from build123d import *

# Parameters (mm, degrees)
SKETCH1_W               = 131
SKETCH1_H               = 106
BOSS_EXTRUDE1_DEPTH     = 5
SKETCH6_R               = 2
CUT_EXTRUDE1_DEPTH      = 4
SKETCH7_R               = 1.4
CUT_EXTRUDE2_DEPTH      = 2.8
MIRROR2_COPY_1_SKETCH_R = 2
MIRROR2_COPY_1_DEPTH    = 4
MIRROR2_COPY_2_SKETCH_R = 1.4
MIRROR2_COPY_2_DEPTH    = 2.8
SKETCH10_W              = 40
SKETCH10_H              = 66
CUT_EXTRUDE5_DEPTH      = 1
FILLET1_R               = 2
SKETCH8_W               = 110
SKETCH8_H               = 99
BOSS_EXTRUDE2_DEPTH     = 1
SKETCH11_W              = 7
SKETCH11_H              = 85
BOSS_EXTRUDE3_DEPTH     = 1


with BuildPart() as part:
    # Sketch1 → Boss-Extrude1 (new body)
    with BuildSketch(Plane.XY):
        with Locations((65.5, 53)):
            Rectangle(SKETCH1_W, SKETCH1_H)
    extrude(amount=BOSS_EXTRUDE1_DEPTH)

    # Sketch6 → Cut-Extrude1 (cut)
    with BuildSketch(Plane(origin=(0, 0, 0), x_dir=(-1, 0, 0), z_dir=(0, 0, -1))):
        with Locations((-5, 5)):
            Circle(SKETCH6_R)
    cut_extrude1 = extrude(amount=-CUT_EXTRUDE1_DEPTH, mode=Mode.SUBTRACT)

    # Sketch7 → Cut-Extrude2 (cut)
    with BuildSketch(Plane(origin=(0, 0, 4), x_dir=(-1, 0, 0), z_dir=(0, 0, -1))):
        with Locations((-5, 5)):
            Circle(SKETCH7_R)
    cut_extrude2 = extrude(amount=-CUT_EXTRUDE2_DEPTH, mode=Mode.SUBTRACT)

    # Mirror1: Cut-Extrude1, Cut-Extrude2 across plane
    add(cut_extrude1.mirror(Plane.ZY.offset(-65.5)), mode=Mode.SUBTRACT)
    add(cut_extrude2.mirror(Plane.ZY.offset(-65.5)), mode=Mode.SUBTRACT)

    # Mirror2: Cut-Extrude1, Cut-Extrude2 across plane
    add(cut_extrude1.mirror(Plane(origin=(0, 53, 0), x_dir=(0, 0, 1), z_dir=(0, -1, 0))), mode=Mode.SUBTRACT)
    add(cut_extrude2.mirror(Plane(origin=(0, 53, 0), x_dir=(0, 0, 1), z_dir=(0, -1, 0))), mode=Mode.SUBTRACT)

    # Mirror2 copy 1 sketch → Mirror2 copy 1 (cut)
    with BuildSketch(Plane(origin=(131, 106, 0), x_dir=(1, 0, 0), z_dir=(0, 0, -1))):
        with Locations((-5, 5)):
            Circle(MIRROR2_COPY_1_SKETCH_R)
    extrude(amount=-MIRROR2_COPY_1_DEPTH, mode=Mode.SUBTRACT)

    # Mirror2 copy 2 sketch → Mirror2 copy 2 (cut)
    with BuildSketch(Plane(origin=(131, 106, 4), x_dir=(1, 0, 0), z_dir=(0, 0, -1))):
        with Locations((-5, 5)):
            Circle(MIRROR2_COPY_2_SKETCH_R)
    extrude(amount=-MIRROR2_COPY_2_DEPTH, mode=Mode.SUBTRACT)

    # Sketch10 → Cut-Extrude5 (cut)
    with BuildSketch(Plane(origin=(0, 0, 0), x_dir=(-1, 0, 0), z_dir=(0, 0, -1))):
        with Locations((-81, 53)):
            Rectangle(SKETCH10_W, SKETCH10_H)
    extrude(amount=-CUT_EXTRUDE5_DEPTH, mode=Mode.SUBTRACT)

    # Fillet1
    fillet1_edges = [part.edges().sort_by_distance(p)[0] for p in [
        (65.5, 106, 0),
        (131, 53, 0),
        (65.5, 0, 0),
        (0, 53, 0),
        (0, 106, 2.5),
        (131, 106, 2.5),
        (131, 0, 2.5),
        (0, 0, 2.5),
    ]]
    fillet(fillet1_edges, radius=FILLET1_R)

    # Sketch8 → Boss-Extrude2 (add)
    with BuildSketch(Plane.XY.offset(5)):
        with Locations((65.5, 53)):
            Rectangle(SKETCH8_W, SKETCH8_H)
    extrude(amount=BOSS_EXTRUDE2_DEPTH)

    # Sketch11 → Boss-Extrude3 (add)
    with BuildSketch(Plane.XY.offset(5)):
        with Locations((7, 53)):
            Rectangle(SKETCH11_W, SKETCH11_H)
    boss_extrude3 = extrude(amount=BOSS_EXTRUDE3_DEPTH)

    # Mirror3: Boss-Extrude3 across plane
    add(boss_extrude3.mirror(Plane.ZY.offset(-65.5)))


solid = part.part
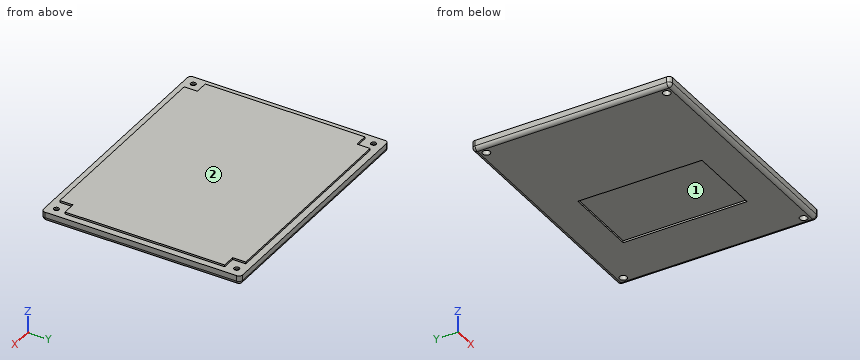
Design review of the part built by this model. Coordinates are the model's own, in mm. Face numbers are marked on the shaded views. Coordinates: 2 decimals unless noted, no trailing zeros. Write each loop counter-clockwise with the first axis right and the second up, starting at its lowest first coordinate (ties: lowest second). Pieces come first, ordered by that corner, then holes. Notation, with made-up numbers: (-8.5, 41.25) -> (44.5, 41.25) arc R20 cw to (44.5, 72.25) -> close; hole circle Ø5 at (10.5, 29.5). An arc over 180 degrees is marked (long way). Write each question's results on one line, items separated by ' | '. Start each with the question number.
(1) For line 1 along Y through (x, z) = (126, 4.6); line 2 along Y through (x, z) = (5, 2.45); line 3 along X through (y, z) = (101, 0.9), list the stretches that pass through material, from the lowest coordinate up. Write a range as from..to.
(2) The part is to be moulded in two halves that separate along Y. For the marked faces 1 and 2, say which applies: pulls with the +Y half, pulls with the -Y half, needs draft (parallel to the pull), parting line crosses it, or undercut.
(3) Clearance check with flat-ended pins moving along their axes: P1, Ø1.7, axis at x = 5, y = 101, coming from the -Z side; P2, Ø0.8, axis at x = 125.5, z = 5.5, coming from the +Y side; P3, Ø0.8, axis at y = 98, z = 5.5, coming from the -X side; P4, Ø0.8, axis at x = 78, z = 5.5, coming from the -Y side. State where each tip first meets the part, or that it passes through.
(4) Take a section at C-C on y = 57.5. Write out the cut boundary in (x, z), and give its area (3 significant figures).
(5) Take a section at A-A on x = 5. Write out the cut boundary in (y, z), and give its area (3 significant figures).
(6) Take a section at B-B on y = 101. Write out the cut boundary in (x, z).
(7) Take a section at D-D on x = 67. Write out the cut boundary in (y, z), and give its area (3 significant figures).
Results found:
1) line 1: y = 0..3.6, 6.4..99.6, 102.4..106 | line 2: y = 0..3, 7..99, 103..106 | line 3: x = 0.33..3, 7..124, 128..130.67
2) face 1: undercut | face 2: needs draft
3) P1: passes through | P2: stops at y = 95.5 | P3: stops at x = 10.5 | P4: stops at y = 3.5
4) outline: (0, 2) arc R2 ccw to (2, 0) -> (61, 0) -> (61, 1) -> (101, 1) -> (101, 0) -> (129, 0) arc R2 ccw to (131, 2) -> (131, 5) -> (127.5, 5) -> (127.5, 6) -> (3.5, 6) -> (3.5, 5) -> (0, 5) -> close | area: 737 mm2
5) outline: (0, 2) arc R2 ccw to (2, 0) -> (3, 0) -> (3, 4) -> (3.6, 4) -> (3.6, 5) -> (0, 5) -> close; (6.4, 4) -> (7, 4) -> (7, 0) -> (99, 0) -> (99, 4) -> (99.6, 4) -> (99.6, 5) -> (95.5, 5) -> (95.5, 6) -> (10.5, 6) -> (10.5, 5) -> (6.4, 5) -> close; (102.4, 4) -> (103, 4) -> (103, 0) -> (104, 0) arc R2 ccw to (106, 2) -> (106, 5) -> (102.4, 5) -> close | area: 576 mm2
6) outline: (0, 2) arc R2 ccw to (2, 0) -> (3, 0) -> (3, 4) -> (3.6, 4) -> (3.6, 5) -> (0, 5) -> close; (6.4, 4) -> (7, 4) -> (7, 0) -> (124, 0) -> (124, 4) -> (124.6, 4) -> (124.6, 5) -> (120.5, 5) -> (120.5, 6) -> (10.5, 6) -> (10.5, 5) -> (6.4, 5) -> close; (127.4, 4) -> (128, 4) -> (128, 0) -> (129, 0) arc R2 ccw to (131, 2) -> (131, 5) -> (127.4, 5) -> close
7) outline: (0, 2) arc R2 ccw to (2, 0) -> (20, 0) -> (20, 1) -> (86, 1) -> (86, 0) -> (104, 0) arc R2 ccw to (106, 2) -> (106, 5) -> (102.5, 5) -> (102.5, 6) -> (3.5, 6) -> (3.5, 5) -> (0, 5) -> close | area: 561 mm2
